Autodesk Inventor part; units mm, degrees
ref_plane "Work Plane1" through (0, 12.7, 0) normal (0, -1, 0) x (1, 0, 0)
ref_plane "YZ Plane" through (0, 0, 0) normal (1, 0, 0) x (0, 1, 0)
ref_plane "XZ Plane" through (0, 0, 0) normal (0, 1, 0) x (-1, 0, 0)
sketch "Sketch1" plane through (0, 0, 0) normal (1, 0, 0) x (0, 1, 0)
  line L0 (0, 0) -> (25.4, 0)
  line L1 (25.4, 0) -> (25.4, -50.8)
  line L2 (25.4, -50.8) -> (0, -50.8)
  line L3 (0, -50.8) -> (0, 0)
  dimension "d0" = 25.4
  dimension "d1" = 50.8
extrude "Extrusion1" add sketch "Sketch1" along normal blind 3.175
sketch "Sketch2" plane through (0, 25.4, 0) normal (0, 1, 0) x (1, 0, 0)
  line L0 (0, 50.8) -> (3.175, 50.8)
  arc A0 (3.175, 53.557) -> (0, 51.8122) centre (-1.9772, 59.1712) ccw
  line L1 (0, 50.8) -> (0, 0)
  line L2 (0, 50.8) -> (0, 51.8122)
  line L3 (3.175, 50.8) -> (3.175, 53.557)
  dimension "d4" = 15.24
extrude "Extrusion2" add sketch "Sketch2" against normal blind 6.35
ref_plane "Work Plane1" through (0, 12.7, 0) normal (0, -1, 0) x (1, 0, 0)
sketch "Sketch3" plane through (0, 12.7, 0) normal (0, -1, 0) x (1, 0, 0)
  arc A0 (0, -51.8122) -> (3.175, -53.557) centre (-1.9772, -59.1712) ccw
  line L0 (3.175, -53.557) -> (3.175, -50.8)
  line L1 (0, -50.8) -> (3.175, -50.8)
  line L2 (0, -50.8) -> (0, -51.8122)
  point P0 (0, 0)
extrude "Extrusion3" add sketch "Sketch3" along normal blind 6.35
sketch "Sketch4" plane through (0, 25.4, 0) normal (0, 1, 0) x (1, 0, 0)
  arc A0 (3.175, 53.557) -> (0, 51.8122) centre (-1.9772, 59.1712) ccw
  circle A1 centre (-1.9772, 59.1712) radius 6.35
  point P0 (0, 0)
  dimension "d10" = 12.7
extrude "Extrusion4" cut sketch "Sketch4" against normal blind 127
sketch "Sketch5" plane through (3.175, 0, 0) normal (1, 0, 0) x (0, 0, -1)
  line L0 (0, 25.4) -> (0, 0) construction
  line L1 (0, 12.7) -> (12.7, 12.7) construction
  line L2 (12.7, 12.7) -> (31.75, 12.7) construction
  circle A0 centre (12.7, 12.7) radius 2.5797
  circle A1 centre (31.75, 12.7) radius 2.5797
  dimension "d13" = 12.7
  dimension "d14" = 19.05
  dimension "d15" = 5.1594
  dimension "d16" = 5.1594
extrude "Extrusion5" cut sketch "Sketch5" against normal blind 127
properties part number "hinge half"
Design review of the part built by this model. Coordinates are the model's own, in mm. A direction names the side the tool comes from. Round coordinates to 2 decimals unless told otherwise and drop trailing zeros. Write each loop counter-clockwise with the first axis right and the second up, starting at its lowest first coordinate (ties: lowest second). Pieces come first, ordered by that corner, then holes. Notation, with made-up numbers: (39, -33.5) -> (60, -33.5) arc R27 cw to (60, -6.5) -> close; hole circle Ø6 at (-38, 28). An arc over 180 degrees is marked (long way). Write item = value, one per line. Start each with the question number.
1) Take a section at A-A, the plane z = -12.7. State the section outline as (x, y) points (3 decimals).
2) Clearance check with flat-ended pins moving along their axes: pin 1 (2.5 mm diameter, centred on x = 1, y = 4, fed in from -Z); pin 2 (3 mm diameter, centred on x = 0, y = 5, fed in from -Z); pin 3 (6 mm diameter, centred on y = 19.5, z = -54, fed in from -X); pin 4 (7.5 mm diameter, centred on x = -5, z = -62.5, fed in from +Y). State where each tip first meets the part, or that it passes through.
3) Take a section at D-D, the plane y = 18. State the section outline as (x, z) points (3 decimals).
4) Mouldability with a two-part tool opening along X and no side actions: class faces 1 (the face through (3.175, 13, -26)), 2 (the face through (-3.35, 22.27, -52.97)), 3 (the face through (1, 12.7, -53)) as +X half, -X half, draft (parallel to the pull), parting line (faces both ways), or undercut.
5) Take a section at C-C, the plane z = -60. State the section outline as (x, y) points.
6) Tool access review of faces 4 (the face through (2, 3, -50.8)), 5 (the face through (2, 16, -50.8)), 6 (the face through (-3.35, 9.57, -52.97)): name each direction out of +Z, -Z, +X, -X, +Y, -Y from which nothing blocks a thin tool from reaching the whole face with its end or side.
7) Take a section at B-B, the plane x = -4.75. State the section outline as (y, z) points, plus the area to 3 significant figures.
8) Wall thickness on probe 1 along Y at (x, z) = (1.7, -31.75); probe 2 along X at (y, z) = (13.5, -47.5) (3 decimals); probe 3 along Z at (x, y) = (1.75, 11.25): over which ranges is each line inside the solid? List them lowest first. Write a range as from..to.
Results list:
q1.outline = (0, 0) -> (3.175, 0) -> (3.175, 10.12) -> (0, 10.12) -> close; (0, 15.28) -> (3.175, 15.28) -> (3.175, 25.4) -> (0, 25.4) -> close
q2.pin_1 = -50.8
q2.pin_2 = -66.68
q2.pin_3 = -9.28
q2.pin_4 = 25.4
q3.outline = (0, -50.8) -> (3.175, -50.8) -> (3.175, 0) -> (0, 0) -> close
q4.face_1 = +X half
q4.face_2 = undercut
q4.face_3 = draft
q5.outline = (-9.55, 6.35) -> (-8.27, 6.35) -> (-8.27, 12.7) -> (-9.55, 12.7) -> close; (-9.55, 19.05) -> (-8.27, 19.05) -> (-8.27, 25.4) -> (-9.55, 25.4) -> close; (4.32, 6.35) -> (5.6, 6.35) -> (5.6, 12.7) -> (4.32, 12.7) -> close; (4.32, 19.05) -> (5.6, 19.05) -> (5.6, 25.4) -> (4.32, 25.4) -> close
q6.face_4 = -Z, +X, -X, -Y
q6.face_5 = -Z, +X, -X
q6.face_6 = +Y, -Y
q7.outline = (6.35, -66.27) -> (12.7, -66.27) -> (12.7, -64.88) -> (6.35, -64.88) -> close; (6.35, -53.46) -> (12.7, -53.46) -> (12.7, -52.07) -> (6.35, -52.07) -> close; (19.05, -66.27) -> (25.4, -66.27) -> (25.4, -64.88) -> (19.05, -64.88) -> close; (19.05, -53.46) -> (25.4, -53.46) -> (25.4, -52.07) -> (19.05, -52.07) -> close
q7.area = 35.2 mm²
q8.probe_1 = 0..10.12, 15.28..25.4
q8.probe_2 = 0..3.175
q8.probe_3 = -65.82..-64.31, -54.03..-33.88, -29.62..-14.83, -10.57..0
